The drawing under review shows one solid part. Ordinate dimensions are in mm from its lowest x, y, z. A direction names the side the tool comes from. Coordinates: 2 decimals unless noted, no trailing zeros. Loops run counter-clockwise (first coordinate to the right, second up) from the corner with the lowest first, then second, coordinate; pieces in that order, holes last. Notation, with made-up numbers: (-38.75, 79.25) - (1.25, 79.25) arc R13 ccw to (1.25, 97.25) - close; hole circle Ø1 at (2, 13.25). An arc over 180 degrees is marked (long way). Answer as a JSON object with one key per item and string values. Group by question number.
Item 1: We need section D-D (y = 8). Give the boundary of the cut face in (x, z).
Item 2: We need section C-C (y = 21.5). Give the boundary of the cut face in (x, z).
Item 3: We need section A-A (z = 31.5). Give the boundary of the cut face in (x, y), then the cut area to 3 significant figures.
Item 4: Clearance check with flat-ended pins moving along their axes: pin 1 (1 mm diameter, centred on y = 57, z = 25.5, fed in from -X); pin 2 (5 mm diameter, centred on x = 47.06, z = 15.94, fed in from +Y); pin 3 (1 mm diameter, centred on y = 45, z = 50.5, fed in from -X) (1 decimal). State where each tip first meets the part, or that it passes through.
Item 5: We need section B-B (x = 31.5). Give the boundary of the cut face in (y, z).
Item 6: To check wall thickness, follow line 1 (Y direction, x = 12, z = 49.5); line 2 (Z direction, x = 60.5, y = 17) (1 decimal); line 3 (X direction, y = 52.5, z = 14.5). State the ranges of each line that lie inside material, in increasing order.
Item 7: Tool access review of the marked faces 1 and 2: name each direction out of +Z, -Z, +X, -X, +Y, -Y from which nothing blocks a thin tool from reaching the whole face with its end or side.
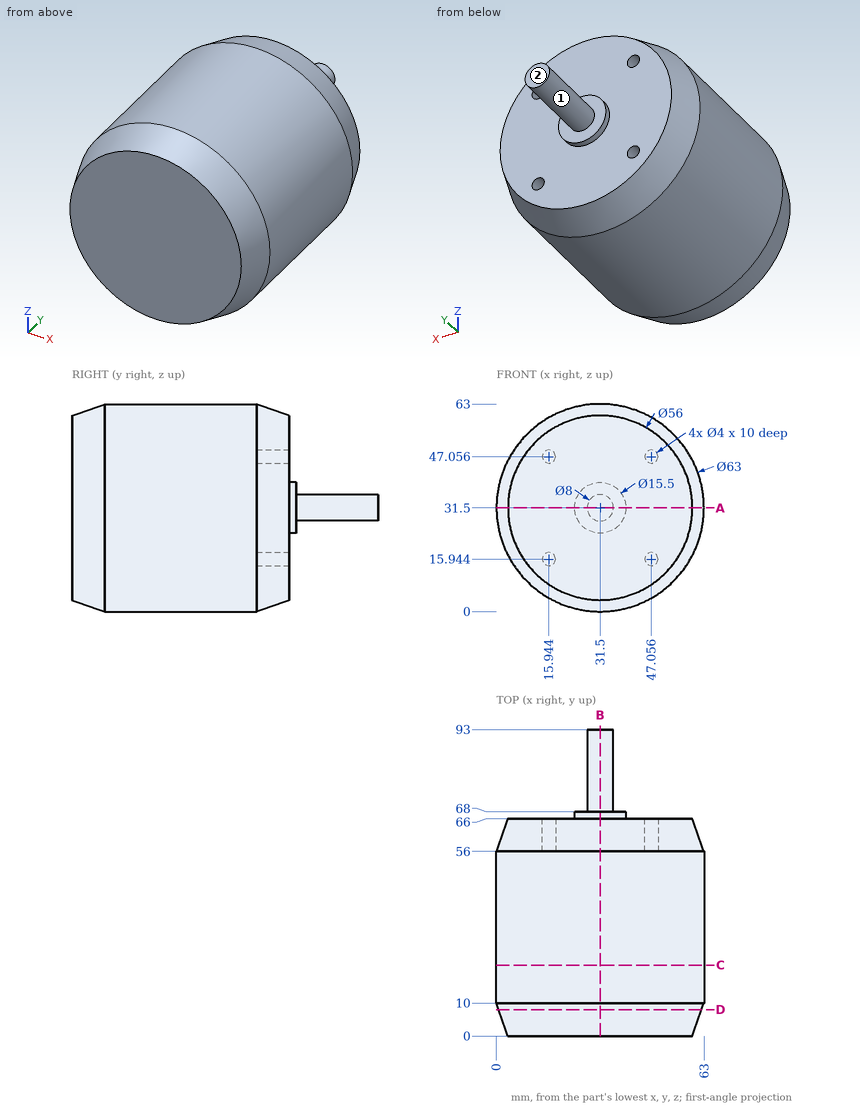
Check sheet entries:
{
 "1": {"outline": "circle Ø61.6 at (31.5, 31.5)"},
 "2": {"outline": "circle Ø63 at (31.5, 31.5)"},
 "3": {"outline": "(0, 10) - (3.5, 0) - (59.5, 0) - (63, 10) - (63, 56) - (59.5, 66) - (39.25, 66) - (39.25, 68) - (35.5, 68) - (35.5, 93) - (27.5, 93) - (27.5, 68) - (23.75, 68) - (23.75, 66) - (3.5, 66) - (0, 56) - close", "area": "4,320 mm2"},
 "4": {"pin 1": "stops at x = 0.73", "pin 2": "stops at y = 66", "pin 3": "stops at x = 6"},
 "5": {"outline": "(0, 3.5) - (10, 0) - (56, 0) - (66, 3.5) - (66, 23.75) - (68, 23.75) - (68, 27.5) - (93, 27.5) - (93, 35.5) - (68, 35.5) - (68, 39.25) - (66, 39.25) - (66, 59.5) - (56, 63) - (10, 63) - (0, 59.5) - close"},
 "6": {"line 1": "y = 0 to 66", "line 2": "z = 19.2 to 43.8", "line 3": "x = 4.98 to 58.02"},
 "7": {"face 1": "+Y", "face 2": "+Z, -Z, +X, -X, +Y"}
}
